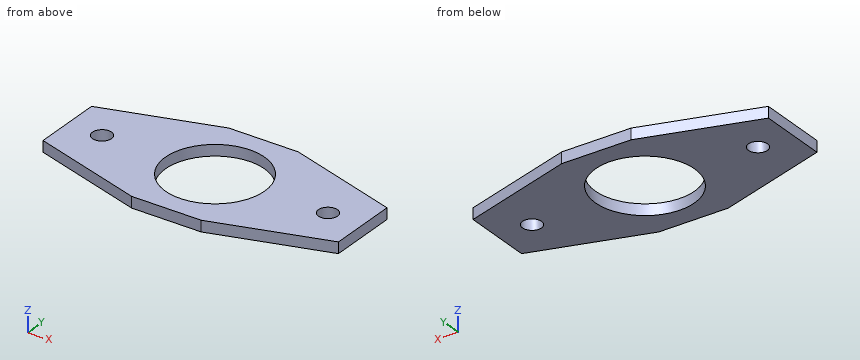
from build123d import *

# Parameters (mm, degrees)
SKETCH1_W           = 85
SKETCH1_H           = 40
BOSS_EXTRUDE1_DEPTH = 3.175
SKETCH2_R           = 14.275
CUT_EXTRUDE1_DEPTH  = 4.175
SKETCH4_OUTSIDE_W   = 105.8
SKETCH4_OUTSIDE_H   = 60.8
CUT_EXTRUDE4_DEPTH  = 4.175
SKETCH6_R           = 2.75
CUT_EXTRUDE6_DEPTH  = 4.175


with BuildPart() as part:
    # Sketch1 → Boss-Extrude1 (new body)
    with BuildSketch(Plane.XY):
        with Locations((42.5, 20)):
            Rectangle(SKETCH1_W, SKETCH1_H)
    extrude(amount=BOSS_EXTRUDE1_DEPTH)

    # Sketch2 → Cut-Extrude1 (cut, through all)
    with BuildSketch(Plane.XY.offset(3.175)):
        with Locations((42.5, 20)):
            Circle(SKETCH2_R)
    extrude(amount=-CUT_EXTRUDE1_DEPTH, mode=Mode.SUBTRACT)

    # Sketch4 outside → Cut-Extrude4 (cut, through all)
    with BuildSketch(Plane(origin=(0, 0, 0), x_dir=(-1, 0, 0), z_dir=(0, 0, -1))):
        with Locations((-42.5, 20)):
            Rectangle(SKETCH4_OUTSIDE_W, SKETCH4_OUTSIDE_H)
        Polygon((-32.5, 40), (0, 30), (0, 10), (-32.5, 0), (-52.5, 0), (-85, 10), (-85, 30), (-52.5, 40), align=None, mode=Mode.SUBTRACT)
    extrude(amount=-CUT_EXTRUDE4_DEPTH, mode=Mode.SUBTRACT)

    # Sketch6 → Cut-Extrude6 (cut, through all)
    with BuildSketch(Plane(origin=(0, 0, 0), x_dir=(-1, 0, 0), z_dir=(0, 0, -1))):
        with Locations((-75, 20)):
            Circle(SKETCH6_R)
        with Locations((-10, 20)):
            Circle(SKETCH6_R)
    extrude(amount=-CUT_EXTRUDE6_DEPTH, mode=Mode.SUBTRACT)


solid = part.part
The model under review builds one solid part; all positions refer to its coordinate system, in mm. Round coordinates to 2 decimals unless told otherwise and drop trailing zeros. Write each loop counter-clockwise with the first axis right and the second up, starting at its lowest first coordinate (ties: lowest second). Pieces come first, ordered by that corner, then holes. Notation, with made-up numbers: (12.25, 15) - (65.25, 15) arc R30 cw to (65.25, 37) - close; hole circle Ø5 at (-19, 67.5). An arc over 180 degrees is marked (long way). One line per item, written item: value. Start each with the question number.
1. To check wall thickness, follow L1, parallel to Y at x = 42.5, z = 1.3 (3 decimals); L2, parallel to X at y = 12.5, z = 1.05; L3, parallel to Y at x = 74.5, z = 0.6. State the ranges of each line that lie inside material, in increasing order. Write a range as from..to.
2. Consider section D-D on y = 25.5. Write out the cut boundary in (x, z) (3 decimals).
3. Consider section A-A on y = 20. Write out the cut boundary in (x, z) (3 decimals), and give its area (3 significant figures).
4. Clearance check with flat-ended pins moving along their axes: P1, Ø1, axis at x = 56, y = 21, coming from the -Z side; P2, Ø1, axis at x = 60.5, z = 1.5, coming from the +Y side. State where each tip first meets the part, or that it passes through.
5. Consider section C-C on z = 1.35. Write out the cut boundary in (x, y) (3 decimals).
6. Consider section B-B on x = 42.5. Write out the cut boundary in (y, z) (3 decimals).
Checks:
1. L1: y = 0..5.725, 34.275..40
1. L2: x = 0..30.35, 54.65..85
1. L3: y = 6.77..17.3, 22.7..33.23
2. outline: (0, 0) - (29.327, 0) - (29.327, 3.175) - (0, 3.175) - close; (55.673, 0) - (85, 0) - (85, 3.175) - (55.673, 3.175) - close
3. outline: (0, 0) - (7.25, 0) - (7.25, 3.175) - (0, 3.175) - close; (12.75, 0) - (28.225, 0) - (28.225, 3.175) - (12.75, 3.175) - close; (56.775, 0) - (72.25, 0) - (72.25, 3.175) - (56.775, 3.175) - close; (77.75, 0) - (85, 0) - (85, 3.175) - (77.75, 3.175) - close
3. area: 144 mm^2
4. P1: passes through
4. P2: stops at y = 37.69
5. outline: (0, 10) - (32.5, 0) - (52.5, 0) - (85, 10) - (85, 30) - (52.5, 40) - (32.5, 40) - (0, 30) - close; hole circle Ø5.5 at (10, 20); hole circle Ø28.55 at (42.5, 20); hole circle Ø5.5 at (75, 20)
6. outline: (0, 0) - (5.725, 0) - (5.725, 3.175) - (0, 3.175) - close; (34.275, 0) - (40, 0) - (40, 3.175) - (34.275, 3.175) - close
